Autodesk Inventor part; units mm, degrees
ref_plane "Work Plane2" through (3, -200, 0) normal (1, 0, 0) x (0, 0, -1)
ref_plane "YZ Plane" through (0, 0, 0) normal (1, 0, 0) x (0, 1, 0)
ref_plane "XZ Plane" through (0, 0, 0) normal (0, 1, 0) x (-1, 0, 0)
ref_plane "Work Plane2" through (3, -200, 0) normal (1, 0, 0) x (0, 0, -1)
sketch "Sketch1" plane through (3, -200, 0) normal (1, 0, 0) x (0, 0, -1)
  circle A0 centre (10, 15) radius 2.5
  circle A1 centre (10, 15) radius 6
  circle A2 centre (44.112, 15) radius 2.5
  circle A3 centre (44.112, 15) radius 6
  circle A4 centre (44.112, 50) radius 2.5
  circle A5 centre (44.112, 50) radius 6
  circle A6 centre (10, 50) radius 2.5
  circle A7 centre (10, 50) radius 6
  circle A8 centre (10, 100) radius 2.5
  circle A9 centre (10, 100) radius 6
  circle A10 centre (44.112, 100) radius 2.5
  circle A11 centre (44.112, 100) radius 6
  circle A12 centre (10, 150) radius 2.5
  circle A13 centre (10, 150) radius 6
  circle A14 centre (44.112, 150) radius 2.5
  circle A15 centre (44.112, 150) radius 6
  circle A16 centre (10, 185) radius 2.5
  circle A17 centre (10, 185) radius 6
  circle A18 centre (44.112, 185) radius 2.5
  circle A19 centre (44.112, 185) radius 6
  circle A20 centre (27.056, 185) radius 1.5
  circle A21 centre (27.056, 185) radius 1.5
  circle A22 centre (27.056, 155) radius 1.5
  circle A23 centre (27.056, 155) radius 1.5
  circle A24 centre (27.056, 120) radius 1.5
  circle A25 centre (27.056, 120) radius 1.5
  circle A26 centre (27.056, 85) radius 1.5
  circle A27 centre (27.056, 85) radius 1.5
  circle A28 centre (27.056, 50) radius 1.5
  circle A29 centre (27.056, 50) radius 1.5
  circle A30 centre (27.056, 15) radius 1.5
  circle A31 centre (27.056, 15) radius 1.5
  line L0 (44.112, 9) -> (50.112, 9)
  line L1 (10, 9) -> (4, 9)
  line L2 (10, 191) -> (4, 191)
  line L3 (44.112, 191) -> (50.112, 191)
  line L4 (4, 191) -> (50.112, 191)
  line L5 (50.112, 191) -> (50.112, 9)
  line L6 (50.112, 9) -> (4, 9)
  line L7 (4, 9) -> (4, 191)
  line L8 (10, 56) -> (4, 56)
  line L9 (10, 44) -> (4, 44)
  line L10 (44.112, 56) -> (50.112, 56)
  line L11 (44.112, 44) -> (50.112, 44)
  line L12 (44.112, 21) -> (50.112, 21)
  line L13 (10, 21) -> (4, 21)
  line L14 (10, 94) -> (4, 94)
  line L15 (10, 106) -> (4, 106)
  line L16 (10, 144) -> (4, 144)
  line L17 (10, 156) -> (4, 156)
  line L18 (44.112, 156) -> (50.112, 156)
  line L19 (44.112, 144) -> (50.112, 144)
  line L20 (44.112, 179) -> (50.112, 179)
  line L21 (10, 179) -> (4, 179)
  line L22 (16, 185) -> (16, 191)
  line L23 (38.112, 185) -> (38.112, 191)
  line L24 (16, 15) -> (16, 9)
  line L25 (38.112, 15) -> (38.112, 9)
  line L26 (44.112, 106) -> (50.112, 106)
  line L27 (44.112, 94) -> (50.112, 94)
  point P0 (0, 200)
  point P1 (50.112, 100)
  dimension "d1" = 12
  dimension "d2" = 12
  dimension "d3" = 12
  dimension "d4" = 12
  dimension "d5" = 12
  dimension "d6" = 12
  dimension "d7" = 12
  dimension "d8" = 12
  dimension "d9" = 12
  dimension "d10" = 12
extrude "Extrusion1" add sketch "Sketch1" along normal blind 5 contours A1 L13 L7 L9 A7 L8 L14 A9 L15 L16 A13 L17 L21 A17 L22 L4 L23 A19 L20 L5 L18 A15 L19 L26 A11 L27 L10 A5 L11 L12 A3 L25 L6 L24
equation "\"BendRadius\" = Thickness"
equation "\"BendReliefWidth\" = Thickness"
equation "\"BendReliefDepth\" = 0.5 * Thickness"
equation "\"CornerReliefSize\" = 4 * Thickness"
equation "\"MinimumRemnant\" = 2 * Thickness"
equation "\"TransitionRadius\" = BendRadius"
equation "\"JacobiRadiusSize\" = BendRadius"
equation "\"GapSize\" = Thickness"
properties part number "linrail_screw_spacer" material "PET Plastic"
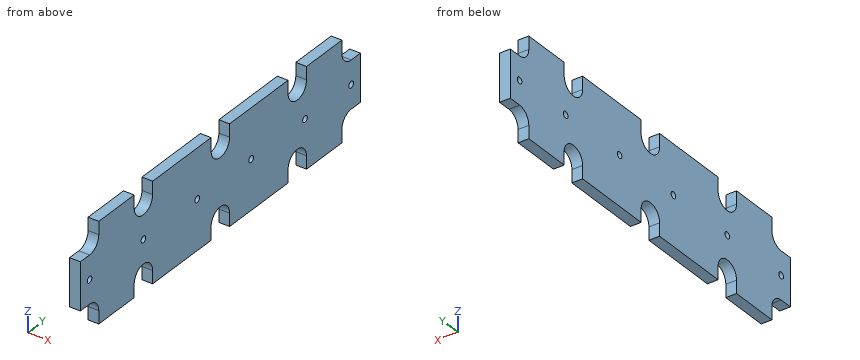
For this review, take the finished solid that the model builds, in its own axes (mm). Round coordinates to 2 decimals unless told otherwise and drop trailing zeros. Order: outer loops, then holes, each group sorted by start corner. A loop starts at its lowest first (then second) coordinate and runs counter-clockwise, first axis right, second up. Notation, with made-up numbers: M 43.25,-10.5 L 57.25,-10.5 A18 ccw 57.25,23.5 Z; hole C -10.75,30 d9. An arc over 180 degrees is marked long. Write each question's results on one line, items separated by ' | '. Start each with the question number.
1. Add section B-B (y = -100). State the section outline as (x, z) points.
2. To check wall thickness, follow L1, parallel to Y at x = 4.7, z = -7.5; L2, parallel to Z at x = 4.8, y = -80; L3, parallel to Z at x = 5.95, y = -150. State the ranges of each line that lie inside material, in increasing order. Write a range as [from, to].
3. Add section A-A (x = 4.45). State how many separate pieces and enclosed holes the cut face has, then the cut area to 3 significant figures.
4. Clearance check with flat-ended pins moving along their axes: pin 1 Ø1 at (x, y) = (5.5, -95.5) entering from +Z; pin 2 Ø1.5 at (x, z) = (4.5, -5.5) entering from +Y; pin 3 Ø1.5 at (x, z) = (4.5, -48) entering from -Y; pin 4 Ø2.5 at (y, z) = (-115, -27.056) entering from -X. State where each tip first meets the part, or that it passes through.
Output values:
1) outline: M 3,-38.11 L 8,-38.11 L 8,-16 L 3,-16 Z
2) L1: [-179, -156], [-144, -106], [-94, -56], [-44, -21] | L2: [-50.11, -28.56], [-25.56, -4] | L3: [-38.11, -28.56], [-25.56, -16]
3) separate pieces: 1 | enclosed holes: 6 | area: 7,030 mm^2
4) pin 1: z = -13.32 | pin 2: y = -21 | pin 3: y = -179 | pin 4: through
